Job drawing, mm, ordinate dimensions from the low corner. One solid piece. A direction names the side the tool comes from. Round coordinates to 2 decimals unless told otherwise and drop trailing zeros. Write each loop counter-clockwise with the first axis right and the second up, starting at its lowest first coordinate (ties: lowest second). Pieces come first, ordered by that corner, then holes. Notation, with made-up numbers: (-40, 56.25) -> (-5, 56.25) arc R21 cw to (-5, 61.25) -> close; hole circle Ø2 at (26.25, -31.5). An arc over 180 degrees is marked (long way). Use CSV: the item, a comma, the result in double quotes. Start each with the question number.
(1) Saw through at A-A (y = 13.25). Give the cut face in (x, z), plus the area to 3 significant figures.
(2) Saw through at D-D (y = 3.5). Give the cut face in (x, z).
(3) Saw through at C-C (z = 2.75). Give the cut face in (x, y).
(4) Drop flat-ended pins along their axis: pin 1 (5 mm diameter, centred on x = 5, y = 5, fed in from +Z); pin 2 (3 mm diameter, centred on y = 16, z = 2.5, fed in from +X); pin 3 (1.5 mm diameter, centred on x = 33, y = 20, fed in from +Z); pin 4 (0.5 mm diameter, centred on x = 22, z = 0.5, fed in from +Y). Give the stop position or say it passes through.
(5) Probe line 1 (X direction, y = 15.75, z = 5.25); line 2 (X direction, y = 2, z = 5.2); line 3 (Y direction, x = 5, z = 4.1). List the from-to ranges inside material, lowest first. Write a range as [from, to].
(6) Two-plate mould, pull along X, no slides. Class the marked faces 4, 5 and 6: released by +X, released by -X, zero draft, split by the parting line, or undercut.
(7) Saw through at B-B (x = 20). Give the cut face in (y, z), plus the area to 3 significant figures.
(8) Which spindle directions (+Z, -Z, +X, -X, +Y, -Y) get a long thin tool onto all of the face, cutting with end or side? Do the marked faces 1, 2 and 3. Say none if no direction does.
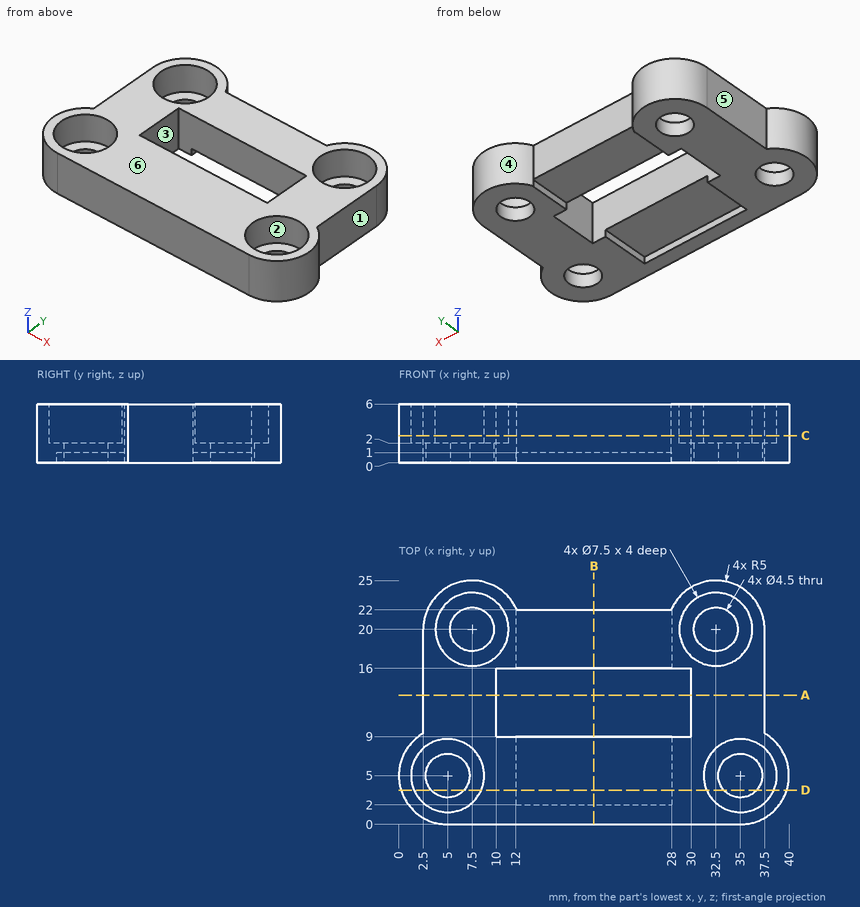
Answers:
1,outline,"(2.5, 0) -> (10, 0) -> (10, 6) -> (2.5, 6) -> close; (30, 0) -> (37.5, 0) -> (37.5, 6) -> (30, 6) -> close"
1,area,"90.0 mm²"
2,outline,"(0.23, 0) -> (3.32, 0) -> (3.32, 2) -> (1.56, 2) -> (1.56, 6) -> (0.23, 6) -> close; (6.68, 0) -> (12, 0) -> (12, 1) -> (28, 1) -> (28, 0) -> (33.32, 0) -> (33.32, 2) -> (31.56, 2) -> (31.56, 6) -> (8.44, 6) -> (8.44, 2) -> (6.68, 2) -> close; (36.68, 0) -> (39.77, 0) -> (39.77, 6) -> (38.44, 6) -> (38.44, 2) -> (36.68, 2) -> close"
3,outline,"(2.5, 9.33) arc R5 ccw to (5, 0) -> (35, 0) arc R5 ccw to (37.5, 9.33) -> (37.5, 20) arc R5 ccw to (27.92, 22) -> (12.08, 22) arc R5 ccw to (2.5, 20) -> close; hole circle Ø7.5 at (5, 5); hole circle Ø7.5 at (7.5, 20); hole (10, 9) -> (30, 9) -> (30, 16) -> (10, 16) -> close; hole circle Ø7.5 at (32.5, 20); hole circle Ø7.5 at (35, 5)"
4,pin 1,"stops at z = 2"
4,pin 2,"stops at x = 37.5"
4,pin 3,"passes through"
4,pin 4,"stops at y = 2"
5,line 1,"x = [2.5, 10], [30, 37.5]"
5,line 2,"x = [1, 2.75], [7.25, 32.75], [37.25, 39]"
5,line 3,"y = [0, 1.25], [8.75, 17.2], [22.8, 24.33]"
6,face 4,"undercut"
6,face 5,"released by -X"
6,face 6,"zero draft"
7,outline,"(0, 0) -> (2, 0) -> (2, 1) -> (9, 1) -> (9, 6) -> (0, 6) -> close; (16, 1) -> (22, 1) -> (22, 6) -> (16, 6) -> close"
7,area,"77.0 mm²"
8,face 1,"+Z, -Z, +X, +Y"
8,face 2,"+Z"
8,face 3,"+Z, -Z"
